Could you check a few things on this model? Use its own coordinates, in mm. Coordinates: 2 decimals unless noted, no trailing zeros. Loops run counter-clockwise (first coordinate to the right, second up) from the corner with the lowest first, then second, coordinate; pieces in that order, holes last. Notation, with made-up numbers: M 22.5,79.5 L 79.5,79.5 A15 cw 79.5,102.5 Z; hole C -30,80 d3. An arc over 180 degrees is marked long. Use one line per item in the form item = value. Start each with the question number.
```python
from build123d import *

# Parameters (mm, degrees)
SKETCH3_W                 = 140
SKETCH3_H                 = 140
BOSS_EXTRUDE1_DEPTH       = 5
CUT_EXTRUDE1_DEPTH        = 5
CIRPATTERN1_COUNT         = 4
CUT_EXTRUDE2_REACH        = 101.121
SKETCH7_R                 = 11
CIRPATTERN2_COUNT         = 4
CIRPATTERN3_START         = -70
CIRPATTERN3_OUTLINE_W     = 140
CIRPATTERN3_OUTLINE_H     = 140
CIRPATTERN3_OUTLINE_R     = 0.9
CIRPATTERN3_OUTLINE_R_2   = 11
CIRPATTERN3_DEPTH         = 5
CIRPATTERN3_START_2       = -135
CIRPATTERN3_2_OUTLINE_W   = 140
CIRPATTERN3_2_OUTLINE_H   = 140
CIRPATTERN3_2_OUTLINE_R   = 0.9
CIRPATTERN3_2_OUTLINE_R_2 = 11
CIRPATTERN3_2_DEPTH       = 5
CIRPATTERN4_START         = 65
CIRPATTERN4_OUTLINE_W     = 140
CIRPATTERN4_OUTLINE_H     = 140
CIRPATTERN4_OUTLINE_R     = 0.9
CIRPATTERN4_OUTLINE_R_2   = 11
CIRPATTERN4_DEPTH         = 5


# Read off the part's stored shape, not the designer's step: CirPattern3, CirPattern4
with BuildPart() as part:
    # Sketch3 → Boss-Extrude1 (new body)
    with BuildSketch(Plane.XY):
        Rectangle(SKETCH3_W, SKETCH3_H)
    extrude(amount=BOSS_EXTRUDE1_DEPTH)

    # Sketch4 → Cut-Extrude1 (cut)
    with BuildSketch(Plane.XY.offset(5)):
        with BuildLine():
            Line((7.583144073, 14.654211885), (52.928932188, 60))
            Line((52.928932188, 60), (-54.688394727, 60))
            Line((-54.688394727, 60), (-7.80758307, 14.53587447))
            ThreePointArc((-7.80758307, 14.53587447), (-0.126862728, 16.499512291), (7.583144073, 14.654211885))
        make_face()
    cut_extrude1 = extrude(amount=-CUT_EXTRUDE1_DEPTH, mode=Mode.SUBTRACT)

    # CirPattern1: Cut-Extrude1 ×4 about axis
    cirpattern1_axis = Axis((0, 0, 0), (0, 0, 1))
    for i in range(1, CIRPATTERN1_COUNT):
        add(cut_extrude1.rotate(cirpattern1_axis, i * 360 / CIRPATTERN1_COUNT), mode=Mode.SUBTRACT)

    # Sketch7 → Cut-Extrude2 (cut, up to next)
    with BuildSketch(Plane.XY.offset(5), mode=Mode.PRIVATE) as cut_extrude2_sk1:
        Circle(SKETCH7_R)
    cut_extrude2_tool1 = extrude(cut_extrude2_sk1.sketch, amount=-CUT_EXTRUDE2_REACH, mode=Mode.PRIVATE) & part.part
    add(cut_extrude2_tool1.solids().sort_by_distance((0, 0, 5))[0], mode=Mode.SUBTRACT)

    # Sketch9 → Ø1.8 (1.8) Diameter Hole1 (revolve, cut)
    with BuildSketch(Plane(origin=(11.313708499, -11.313708499, 5), x_dir=(0, -1, 0), z_dir=(1, 0, 0))):
        Polygon((0, 0), (0, 6.540774557), (0.9, 6), (0.9, 0), align=None)
    f_1_8_1_8_diameter_hole1 = revolve(axis=Axis((11.313708499, -11.313708499, 11.35), (0, 0, -1)), mode=Mode.SUBTRACT)

    # CirPattern2: Ø1.8 (1.8) Diameter Hole1 ×4 about axis
    cirpattern2_axis = Axis((0, 0, 0), (0, 0, 1))
    for i in range(1, CIRPATTERN2_COUNT):
        add(f_1_8_1_8_diameter_hole1.rotate(cirpattern2_axis, i * 360 / CIRPATTERN2_COUNT), mode=Mode.SUBTRACT)


with BuildPart() as body_2:
    # CirPattern3 outline → CirPattern3 (new body)
    with BuildSketch(Plane.YZ.offset(CIRPATTERN3_START)):
        with Locations((0, -65)):
            Rectangle(CIRPATTERN3_OUTLINE_W, CIRPATTERN3_OUTLINE_H)
        with BuildLine():
            ThreePointArc((-7.80758307, -79.53587447), (-0.126862728, -81.499512291), (7.583144073, -79.654211885))
            Line((7.583144073, -79.654211885), (52.928932188, -125))
            Line((52.928932188, -125), (-54.688394727, -125))
            Line((-54.688394727, -125), (-7.80758307, -79.53587447))
        make_face(mode=Mode.SUBTRACT)
        with Locations((-11.313708499, -76.313708499)):
            Circle(CIRPATTERN3_OUTLINE_R, mode=Mode.SUBTRACT)
        with Locations((11.313708499, -76.313708499)):
            Circle(CIRPATTERN3_OUTLINE_R, mode=Mode.SUBTRACT)
        with BuildLine():
            Line((60, -12.071067812), (60, -119.688394727))
            Line((60, -119.688394727), (14.53587447, -72.80758307))
            ThreePointArc((14.53587447, -72.80758307), (16.499512291, -65.126862728), (14.654211885, -57.416855927))
            Line((14.654211885, -57.416855927), (60, -12.071067812))
        make_face(mode=Mode.SUBTRACT)
        with BuildLine():
            ThreePointArc((-14.53587447, -57.19241693), (-16.499512291, -64.873137272), (-14.654211885, -72.583144073))
            Line((-14.654211885, -72.583144073), (-60, -117.928932188))
            Line((-60, -117.928932188), (-60, -10.311605273))
            Line((-60, -10.311605273), (-14.53587447, -57.19241693))
        make_face(mode=Mode.SUBTRACT)
        with Locations((-11.313708499, -53.686291501)):
            Circle(CIRPATTERN3_OUTLINE_R, mode=Mode.SUBTRACT)
        with Locations((0, -65)):
            Circle(CIRPATTERN3_OUTLINE_R_2, mode=Mode.SUBTRACT)
        with Locations((11.313708499, -53.686291501)):
            Circle(CIRPATTERN3_OUTLINE_R, mode=Mode.SUBTRACT)
        with BuildLine():
            ThreePointArc((7.80758307, -50.46412553), (0.126862728, -48.500487709), (-7.583144073, -50.345788115))
            Line((-7.583144073, -50.345788115), (-52.928932188, -5))
            Line((-52.928932188, -5), (54.688394727, -5))
            Line((54.688394727, -5), (7.80758307, -50.46412553))
        make_face(mode=Mode.SUBTRACT)
    extrude(amount=CIRPATTERN3_DEPTH)


with BuildPart() as body_3:
    # CirPattern3 2 outline → CirPattern3 2 (new body)
    with BuildSketch(Plane.XY.offset(CIRPATTERN3_START_2)):
        Rectangle(CIRPATTERN3_2_OUTLINE_W, CIRPATTERN3_2_OUTLINE_H)
        with BuildLine():
            Line((52.928932188, -60), (-54.688394727, -60))
            Line((-54.688394727, -60), (-7.80758307, -14.53587447))
            ThreePointArc((-7.80758307, -14.53587447), (-0.126862728, -16.499512291), (7.583144073, -14.654211885))
            Line((7.583144073, -14.654211885), (52.928932188, -60))
        make_face(mode=Mode.SUBTRACT)
        with Locations((-11.313708499, -11.313708499)):
            Circle(CIRPATTERN3_2_OUTLINE_R, mode=Mode.SUBTRACT)
        with Locations((11.313708499, -11.313708499)):
            Circle(CIRPATTERN3_2_OUTLINE_R, mode=Mode.SUBTRACT)
        with BuildLine():
            ThreePointArc((14.53587447, -7.80758307), (16.499512291, -0.126862728), (14.654211885, 7.583144073))
            Line((14.654211885, 7.583144073), (60, 52.928932188))
            Line((60, 52.928932188), (60, -54.688394727))
            Line((60, -54.688394727), (14.53587447, -7.80758307))
        make_face(mode=Mode.SUBTRACT)
        with BuildLine():
            ThreePointArc((-14.53587447, 7.80758307), (-16.499512291, 0.126862728), (-14.654211885, -7.583144073))
            Line((-14.654211885, -7.583144073), (-60, -52.928932188))
            Line((-60, -52.928932188), (-60, 54.688394727))
            Line((-60, 54.688394727), (-14.53587447, 7.80758307))
        make_face(mode=Mode.SUBTRACT)
        with Locations((-11.313708499, 11.313708499)):
            Circle(CIRPATTERN3_2_OUTLINE_R, mode=Mode.SUBTRACT)
        Circle(CIRPATTERN3_2_OUTLINE_R_2, mode=Mode.SUBTRACT)
        with Locations((11.313708499, 11.313708499)):
            Circle(CIRPATTERN3_2_OUTLINE_R, mode=Mode.SUBTRACT)
        with BuildLine():
            Line((-52.928932188, 60), (54.688394727, 60))
            Line((54.688394727, 60), (7.80758307, 14.53587447))
            ThreePointArc((7.80758307, 14.53587447), (0.126862728, 16.499512291), (-7.583144073, 14.654211885))
            Line((-7.583144073, 14.654211885), (-52.928932188, 60))
        make_face(mode=Mode.SUBTRACT)
    extrude(amount=CIRPATTERN3_2_DEPTH)


with BuildPart() as body_4:
    # CirPattern4 outline → CirPattern4 (new body)
    with BuildSketch(Plane(origin=(0, 0, 0), x_dir=(1, 0, 0), z_dir=(0, 1, 0)).offset(CIRPATTERN4_START)):
        with Locations((0, 65)):
            Rectangle(CIRPATTERN4_OUTLINE_W, CIRPATTERN4_OUTLINE_H)
        with BuildLine():
            Line((-60, 10.311605273), (-60, 117.928932188))
            Line((-60, 117.928932188), (-14.654211885, 72.583144073))
            ThreePointArc((-14.654211885, 72.583144073), (-16.499512291, 64.873137272), (-14.53587447, 57.19241693))
            Line((-14.53587447, 57.19241693), (-60, 10.311605273))
        make_face(mode=Mode.SUBTRACT)
        with Locations((-11.313708499, 53.686291501)):
            Circle(CIRPATTERN4_OUTLINE_R, mode=Mode.SUBTRACT)
        with BuildLine():
            Line((54.688394727, 5), (-52.928932188, 5))
            Line((-52.928932188, 5), (-7.583144073, 50.345788115))
            ThreePointArc((-7.583144073, 50.345788115), (0.126862728, 48.500487709), (7.80758307, 50.46412553))
            Line((7.80758307, 50.46412553), (54.688394727, 5))
        make_face(mode=Mode.SUBTRACT)
        with Locations((11.313708499, 53.686291501)):
            Circle(CIRPATTERN4_OUTLINE_R, mode=Mode.SUBTRACT)
        with Locations((-11.313708499, 76.313708499)):
            Circle(CIRPATTERN4_OUTLINE_R, mode=Mode.SUBTRACT)
        with BuildLine():
            Line((-54.688394727, 125), (52.928932188, 125))
            Line((52.928932188, 125), (7.583144073, 79.654211885))
            ThreePointArc((7.583144073, 79.654211885), (-0.126862728, 81.499512291), (-7.80758307, 79.53587447))
            Line((-7.80758307, 79.53587447), (-54.688394727, 125))
        make_face(mode=Mode.SUBTRACT)
        with Locations((0, 65)):
            Circle(CIRPATTERN4_OUTLINE_R_2, mode=Mode.SUBTRACT)
        with Locations((11.313708499, 76.313708499)):
            Circle(CIRPATTERN4_OUTLINE_R, mode=Mode.SUBTRACT)
        with BuildLine():
            Line((60, 119.688394727), (60, 12.071067812))
            Line((60, 12.071067812), (14.654211885, 57.416855927))
            ThreePointArc((14.654211885, 57.416855927), (16.499512291, 65.126862728), (14.53587447, 72.80758307))
            Line((14.53587447, 72.80758307), (60, 119.688394727))
        make_face(mode=Mode.SUBTRACT)
    extrude(amount=CIRPATTERN4_DEPTH)


with BuildPart() as part_1:
    add(part.part)

    # Combine1: union body 4, body 3, body 2
    add(body_4.part)
    add(body_3.part)
    add(body_2.part)


solid = part_1.part
```
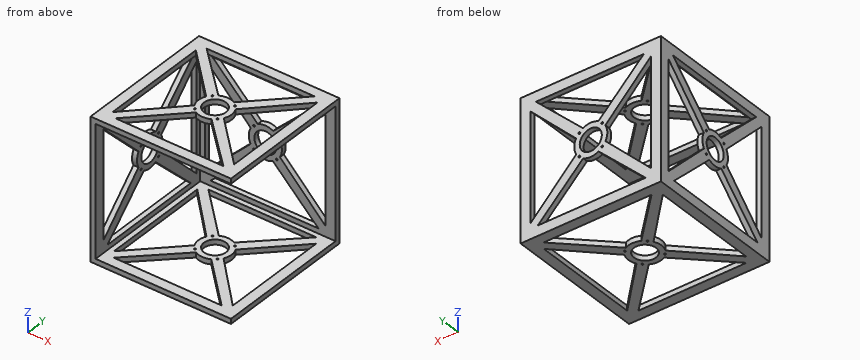
Item 1: I want a section at B-B (z = -123). Write out the boundary of the cut face in (x, y), plus the area to 3 significant figures.
Item 2: Please list where these lines run through material, in increasing order: line 1 along Z through (x, y) = (-27.5, -32.5); line 2 along Z through (x, y) = (-67.05, 0); line 3 along Y through (x, z) = (27, -96.5).
Item 3: I'm going to push flat-ended pins straight in: P1, Ø8, axis at x = 0, z = -56, coming from the +Y side; P2, Ø3, axis at x = 11, z = -55, coming from the -Y side. Where does each tip first touch, or does it pass through?
Item 4: I want a section at A-A (z = -65). Count the separate pieces of the cut face and the enclosed holes in it, plus the area to 3 significant figures.
Worked answers:
q1.outline = M -70,-70 L -65,-70 L -65,-52.63 L -70,-52.63 Z; M -70,50.93 L -65,50.93 L -65,65 L -52.63,65 L -52.63,70 L -70,70 Z; M 50.93,65 L 70,65 L 70,70 L 50.93,70 Z
q1.area = 339 mm²
q2.line_1 = -135 to -130, 0 to 5
q2.line_2 = -135 to -125, -81.5 to -76, -54 to -48.5, -5 to 5
q2.line_3 = 65 to 70
q3.P1 = 70
q3.P2 = 65
q4.separate_pieces = 7
q4.enclosed_holes = 0
q4.area = 285 mm²
